Source: CAD feature listing. Evaluate the final solid. Frame: model axes, mm. A direction names the side the tool comes from. Give positions to 0.01 mm unless a question says otherwise; leave off trailing zeros. Write each loop counter-clockwise with the first axis right and the second up, starting at its lowest first coordinate (ties: lowest second). Pieces come first, ordered by that corner, then holes. Notation, with made-up numbers: (-1, -16.75) -> (10, -16.75) arc R28 ccw to (10, 9.25) -> close; hole circle Ø7 at (38, 26.25). An arc over 180 degrees is marked (long way). Answer as a JSON object with one key per item and string values. Group by question number.
Item 1: Access query for faces 4 (the face through (-113.56, -43.57, 0.3)), 5 (the face through (102.5, -24.6, 0.3)), 6 (the face through (113.464, -43.287, 0.296)), 7 (the face through (-2, -55, 0)). Directions: +Z, -Z, +X, -X, +Y, -Y. A direction counts if a zero-diameter tool reaches every point of the face in a straight line with its end or side. Return the directions, or none.
Item 2: Pull-direction query (X, two-part tool) for faces 1 (the face through (-50.68, -9.16, 0.3)), 2 (the face through (-102.63, -24.77, 0.3)), 3 (the face through (99.358, -78.667, 0.296)); classes: pulls with the +X half, pulls with the -X half, needs draft (parallel to the pull), parting line crosses it, or undercut.
Item 3: Section query A-A on z = 0.5. Give the number of separate pieces and of enclosed holes in the cut face, plus the area to 3 significant figures.
Item 4: Section query B-B on y = -63.5. Return the cut outline in (x, z), plus the area to 3 significant figures.
Item 5: Section query C-C on x = 77.5. Return the cut outline in (y, z), plus the area to 3 significant figures.
Item 6: Ray query, probe 1 along X at (y, z) = (-26, 0.35); probe 2 along Y at (x, z) = (41, 0.5); probe 3 along Y at (x, z) = (21, 0.55). Return the intervals inside material, ascending. Write a range as from..to.
from build123d import *

# Parameters (mm, degrees)
MAIN_SHAPE_DEPTH    = 0.6
TABS_DEPTH          = 154.060061459
TABS_DEPTH_BACK     = 154.060061459
SKETCH4_W           = 90
SKETCH4_H           = 1
TAB_FOLD_LINE_DEPTH = 0.2
CHIN_GUARD_DEPTH    = 0.6
FILLET1_R           = 20


with BuildPart() as part:
    # Sketch1 → Main Shape (new body)
    with BuildSketch(Plane.XY):
        with BuildLine():
            Line((-24, -91.764766734), (24, -91.764766734))
            Line((24, -91.764766734), (78.266232563, -84.05670244))
            ThreePointArc((78.266232563, -84.05670244), (97.655491519, -79.289252293), (115.711102551, -70.764766734))
            ThreePointArc((115.711102551, -70.764766734), (120.685143325, -65.658407438), (122.5, -58.764766734))
            ThreePointArc((122.5, -58.764766734), (120.227482046, -43.118277124), (113.597722286, -28.764766734))
            ThreePointArc((113.597722286, -28.764766734), (107.811505455, -22.955172168), (100.180351554, -19.955641477))
            Line((100.180351554, -19.955641477), (60.74391922, -13.264766734))
            ThreePointArc((60.74391922, -13.264766734), (50.804108255, -9.246591688), (43.461443341, -1.434367632))
            ThreePointArc((43.461443341, -1.434367632), (36.448172688, 5.805997675), (26.941855461, 9.15842781))
            Line((26.941855461, 9.15842781), (17, 10.235233266))
            Line((17, 10.235233266), (10, 0))
            Line((10, 0), (-10, 0))
            Line((-10, 0), (-17, 10.235233266))
            Line((-17, 10.235233266), (-26.941855461, 9.15842781))
            ThreePointArc((-26.941855461, 9.15842781), (-36.448172688, 5.805997675), (-43.461443341, -1.434367632))
            ThreePointArc((-43.461443341, -1.434367632), (-50.804108255, -9.246591688), (-60.74391922, -13.264766734))
            Line((-60.74391922, -13.264766734), (-100.180351554, -19.955641477))
            ThreePointArc((-100.180351554, -19.955641477), (-107.811505455, -22.955172168), (-113.597722286, -28.764766734))
            ThreePointArc((-113.597722286, -28.764766734), (-120.227482046, -43.118277124), (-122.5, -58.764766734))
            ThreePointArc((-122.5, -58.764766734), (-120.685143325, -65.658407438), (-115.711102551, -70.764766734))
            ThreePointArc((-115.711102551, -70.764766734), (-97.655491519, -79.289252293), (-78.266232563, -84.05670244))
            Line((-78.266232563, -84.05670244), (-24, -91.764766734))
        make_face()
    extrude(amount=MAIN_SHAPE_DEPTH)

    # Sketch2 → Tabs (cut, two sides: drawn at the far end of the back side and taken through both)
    with BuildSketch(Plane.XY.offset(0.6).offset(-TABS_DEPTH_BACK)):
        with BuildLine():
            Line((-121, -58.764766734), (-121, -56.764766734))
            Line((-121, -56.764766734), (-115.742268041, -53.771413729))
            ThreePointArc((-115.742268041, -53.771413729), (-113.511139955, -43.427720083), (-109.089826236, -33.814088314))
            Line((-109.089826236, -33.814088314), (-111.5, -28.264766734))
            Line((-111.5, -28.264766734), (-110.3, -26.664766734))
            Line((-110.3, -26.664766734), (-108.3, -25.664766734))
            Line((-108.3, -25.664766734), (-106.7, -26.864766734))
            Line((-106.7, -26.864766734), (-107.9, -28.464766734))
            Line((-107.9, -28.464766734), (-106.3, -29.664766734))
            Line((-106.3, -29.664766734), (-98.84870892, -19.729711961))
            Line((-98.84870892, -19.729711961), (-100.180351554, -19.955641477))
            ThreePointArc((-100.180351554, -19.955641477), (-107.811505455, -22.955172168), (-113.597722286, -28.764766734))
            ThreePointArc((-113.597722286, -28.764766734), (-120.227482046, -43.118277124), (-122.5, -58.764766734))
            ThreePointArc((-122.5, -58.764766734), (-120.767844146, -65.510135516), (-116, -70.586357152))
            Line((-116, -70.586357152), (-116, -58.764766734))
            Line((-116, -58.764766734), (-118, -58.764766734))
            Line((-118, -58.764766734), (-118, -60.764766734))
            Line((-118, -60.764766734), (-120, -60.764766734))
            Line((-120, -60.764766734), (-121, -58.764766734))
        make_face()
        with BuildLine():
            Line((110.3, -26.664766734), (111.5, -28.264766734))
            Line((111.5, -28.264766734), (109.089826236, -33.814088314))
            ThreePointArc((109.089826236, -33.814088314), (113.511139955, -43.427720083), (115.742268041, -53.771413729))
            Line((115.742268041, -53.771413729), (121, -56.764766734))
            Line((121, -56.764766734), (121, -58.764766734))
            Line((121, -58.764766734), (120, -60.764766734))
            Line((120, -60.764766734), (118, -60.764766734))
            Line((118, -60.764766734), (118, -58.764766734))
            Line((118, -58.764766734), (116, -58.764766734))
            Line((116, -58.764766734), (116, -70.586357152))
            ThreePointArc((116, -70.586357152), (120.767844146, -65.510135516), (122.5, -58.764766734))
            ThreePointArc((122.5, -58.764766734), (120.227482046, -43.118277124), (113.597722286, -28.764766734))
            ThreePointArc((113.597722286, -28.764766734), (107.811505455, -22.955172168), (100.180351554, -19.955641477))
            Line((100.180351554, -19.955641477), (98.84870892, -19.729711961))
            Line((98.84870892, -19.729711961), (106.3, -29.664766734))
            Line((106.3, -29.664766734), (107.9, -28.464766734))
            Line((107.9, -28.464766734), (106.7, -26.864766734))
            Line((106.7, -26.864766734), (108.3, -25.664766734))
            Line((108.3, -25.664766734), (110.3, -26.664766734))
        make_face()
    extrude(amount=TABS_DEPTH + TABS_DEPTH_BACK, mode=Mode.SUBTRACT)

    # Sketch4 → Tab Fold Line (cut)
    with BuildSketch(Plane.XY.offset(0.6)):
        with Locations((0, 0.5)):
            Rectangle(SKETCH4_W, SKETCH4_H)
    extrude(amount=-TAB_FOLD_LINE_DEPTH, mode=Mode.SUBTRACT)

    # Sketch5 → Chin guard (add)
    with BuildSketch(Plane.XY.offset(0.6)):
        Polygon((-78.266232563, -84.05670244), (-24, -121.764766734), (24, -121.764766734), (78.266232563, -84.05670244), (24, -91.764766734), (-24, -91.764766734), align=None)
    extrude(amount=-CHIN_GUARD_DEPTH)

    # Fillet1
    fillet1_edges = [part.edges().sort_by_distance(p)[0] for p in [
        (-24, -121.764766734, 0.3),
        (24, -121.764766734, 0.3),
        (78.266232563, -84.05670244, 0.3),
        (-78.266232563, -84.05670244, 0.3),
    ]]
    fillet(fillet1_edges, radius=FILLET1_R)


solid = part.part
Worked answers:
{
 "1": {"face 4": "+Z, -Z, -X", "face 5": "+Z, -Z, +Y", "face 6": "+Z, -Z, +X", "face 7": "-Z, +X, -X, +Y, -Y"},
 "2": {"face 1": "pulls with the -X half", "face 2": "undercut", "face 3": "pulls with the +X half"},
 "3": {"separate pieces": "3", "enclosed holes": "0", "area": "20,700 mm^2"},
 "4": {"outline": "(-116, 0) -> (116, 0) -> (116, 0.6) -> (-116, 0.6) -> close", "area": "139 mm^2"},
 "5": {"outline": "(-84.94, 0) -> (-16.11, 0) -> (-16.11, 0.6) -> (-84.94, 0.6) -> close", "area": "41.3 mm^2"},
 "6": {"probe 1": "-108.97..-107.85, -103.55..103.55, 107.85..108.97", "probe 2": "-109.95..0, 1..1.92", "probe 3": "-121.5..0, 1..9.8"}
}
